Part model, mm, in its own coordinate system. A direction names the side the tool comes from. Round coordinates to 2 decimals unless told otherwise and drop trailing zeros. Write each loop counter-clockwise with the first axis right and the second up, starting at its lowest first coordinate (ties: lowest second). Pieces come first, ordered by that corner, then holes. Notation, with made-up numbers: M 39.25,48.25 L 85.25,48.25 A14 ccw 85.25,73.25 Z; hole C 45,25 d7. An arc over 180 degrees is marked long. Answer as a JSON object with one key per item and string values. Group by question number.
1. Which spindle directions (+Z, -Z, +X, -X, +Y, -Y) get a long thin tool onto all of the face, cutting with end or side? Do faces 5 (the face through (0, 0, 0)), 6 (the face through (0.321, -12.521, 0.947)), 7 (the face through (-3, -5, 0)). Say none if no direction does.
2. Band-saw the part on A-A, the plane y = -6. Write the cut outline in (x, z).
3. Drill centre lines: line 1 (Z direction, x = -1.5, y = -11.25); line 2 (Y direction, x = -2.25, z = 3.25); line 3 (Z direction, x = -2.25, y = -6.75). Where is each one in solid material? Low to high. Write a range as from..to.
4. Band-saw the part on B-B, the plane z = 3.75. Write the cut outline in (x, y).
5. Two-plate mould, pull along X, no slides. Class faces 1 (the face through (1.976, -10.798, -2.258)), 2 (the face through (1.12, -11.036, -1.705)), 3 (the face through (-1, -10, -3)), 4 (the face through (0.66, -12.52, -0.75)): +X half, -X half, draft (parallel to the pull), parting line (faces both ways), or undercut.
6. Drop a flat-ended pin along its axis: pin 1 (4 mm diameter, centred on y = -3, z = -1, fed in from +X). Give the stop position or say it passes through.
from build123d import *

# Parameters (mm, degrees)
F0_R            = 3
F1_DEPTH        = 10
F3_DEPTH        = 5
F5_R            = 1.5
F6_DEPTH        = 2
F6_COPIES_COUNT = 3
F7_R            = 0.25


# Not quite as in the source:
# - a pattern or mirror of a feature is missing from the dataset's text; its kind, count and spacing are read off the source's solid


with BuildPart() as f1:
    # F0 (on Front) → F1 (new body)
    with BuildSketch(Plane.XZ):
        Circle(F0_R)
    extrude(amount=F1_DEPTH)

    # F2 (on face) → F3 (join)
    with BuildSketch(Plane.XZ.offset(10)):
        Polygon((5.858499572, 1.2953697407), (-4.0510728887, 4.4259245871), (-1.8074266833, -5.7212943277), align=None)
    extrude(amount=F3_DEPTH)

    # F5 (on face) → F6 (cut)
    with BuildSketch(Plane(origin=(2.0255364444, 0, -2.2129622935), x_dir=(0.7376540978, 0, 0.6751788148), z_dir=(0.6751788148, 0, -0.7376540978))):
        with Locations((0, 12.5)):
            Circle(F5_R)
    f6 = extrude(amount=-F6_DEPTH, mode=Mode.SUBTRACT)

    # F6_copies: F6 ×3 about axis
    f6_copies_axis = Axis((0, 0, 0), (0, 1, 0))
    for i in range(1, F6_COPIES_COUNT):
        add(f6.rotate(f6_copies_axis, i * 360 / F6_COPIES_COUNT), mode=Mode.SUBTRACT)

    # F7
    f7_edges = [f1.edges().sort_by_distance(p)[0] for p in [
        (5.8585, -12.5, 1.29537),
        (-4.051073, -12.5, 4.425925),
        (-1.807427, -12.5, -5.721294),
    ]]
    fillet(f7_edges, radius=F7_R)


solid = f1.part
Worked answers:
{
 "1": {"face 5": "+Z, -Z, +X, -X, +Y", "face 6": "none", "face 7": "+Y"},
 "2": {"outline": "C 0,0 d6"},
 "3": {"line 1": "z = -5.44..-1.18, 0.52..3.62", "line 2": "y = -15..-10", "line 3": "z = -1.98..1.98"},
 "4": {"outline": "M -3.9,-15 L -1.91,-15 L -1.91,-10 L -3.9,-10 Z"},
 "5": {"face 1": "+X half", "face 2": "undercut", "face 3": "draft", "face 4": "undercut"},
 "6": {"pin 1": "stops at x = 3"}
}
